```python
from build123d import *

# Parameters (mm, degrees)
BASE_EXTRUDE_DEPTH  = 20.447
CUT_EXTRUDE1_DEPTH  = 28.194
SKETCH3_W           = 5.4864
SKETCH3_H           = 1.651
BOSS_EXTRUDE1_DEPTH = 1.27


with BuildPart() as part:
    # Sketch1 → Base-Extrude (new, symmetric)
    with BuildSketch(Plane(origin=(0, 0, 0), x_dir=(1, 0, 0), z_dir=(0, 1, 0))):
        with BuildLine():
            Line((-18.4785, 20.955), (18.4785, 20.955))
            ThreePointArc((18.4785, 20.955), (24.585074162, 18.425574162), (27.1145, 12.319))
            Line((27.1145, 12.319), (27.1145, -12.319))
            ThreePointArc((27.1145, -12.319), (24.585074162, -18.425574162), (18.4785, -20.955))
            Line((18.4785, -20.955), (-18.4785, -20.955))
            ThreePointArc((-18.4785, -20.955), (-24.585074162, -18.425574162), (-27.1145, -12.319))
            Line((-27.1145, -12.319), (-27.1145, 12.319))
            ThreePointArc((-27.1145, 12.319), (-24.585074162, 18.425574162), (-18.4785, 20.955))
        make_face()
    extrude(amount=BASE_EXTRUDE_DEPTH, both=True)

    # Sketch2 → Cut-Extrude1 (cut)
    with BuildSketch(Plane.XZ.offset(20.447)):
        with BuildLine():
            Line((12.192, 20.955), (12.192, -20.955))
            Line((12.192, -20.955), (18.4785, -20.955))
            ThreePointArc((18.4785, -20.955), (24.585074162, -18.425574162), (27.1145, -12.319))
            Line((27.1145, -12.319), (27.1145, 12.319))
            ThreePointArc((27.1145, 12.319), (24.585074162, 18.425574162), (18.4785, 20.955))
            Line((18.4785, 20.955), (12.192, 20.955))
        make_face()
        with BuildLine():
            Line((-18.4785, -20.955), (-12.192, -20.955))
            Line((-12.192, -20.955), (-12.192, 20.955))
            Line((-12.192, 20.955), (-18.4785, 20.955))
            ThreePointArc((-18.4785, 20.955), (-24.585074162, 18.425574162), (-27.1145, 12.319))
            Line((-27.1145, 12.319), (-27.1145, -12.319))
            ThreePointArc((-27.1145, -12.319), (-24.585074162, -18.425574162), (-18.4785, -20.955))
        make_face()
    extrude(amount=-CUT_EXTRUDE1_DEPTH, mode=Mode.SUBTRACT)

    # Sketch3 → Boss-Extrude1 (add)
    with BuildSketch(Plane.XZ.offset(20.447)):
        with Locations((9.4488, -10.4775)):
            Rectangle(SKETCH3_W, SKETCH3_H)
        with Locations((9.4488, 10.4775)):
            Rectangle(SKETCH3_W, SKETCH3_H)
        with Locations((-9.4488, 10.4775)):
            Rectangle(SKETCH3_W, SKETCH3_H)
        with Locations((-9.4488, -10.4775)):
            Rectangle(SKETCH3_W, SKETCH3_H)
    extrude(amount=BOSS_EXTRUDE1_DEPTH)


solid = part.part
```
Geometry: final body of the model. Coordinates: model frame, mm. A direction names the side the tool comes from. Round coordinates to 2 decimals unless told otherwise and drop trailing zeros. Order: outer loops, then holes, each group sorted by start corner. A loop starts at its lowest first (then second) coordinate and runs counter-clockwise, first axis right, second up. Notation, with made-up numbers: (80, 83) -> (126, 83) arc R20 ccw to (126, 122) -> close; hole circle Ø4 at (38.25, 63). An arc over 180 degrees is marked (long way). Use one line per item in the form item = value. Start each with the question number.
1. Cut plane B-B (x = -11). Return the cut outline in (y, z) (3 decimals).
2. Draft query along Z for faces 6 (the face through (-24.65, 14.19, -18.36)), 7 (the face through (20, 7.747, 0)), 8 (the face through (-9, -21, -9.652)). Return one class per face: pulls with the +Z half, pulls with the -Z half, needs draft (parallel to the pull), parting line crosses it, or undercut.
3. Pin query (flat end, axial travel): pin 1 Ø1 at (x, y) = (10, -21) entering from -Z; pin 2 Ø19.5 at (x, z) = (3, -5.5) entering from -Y; pin 3 Ø5 at (x, z) = (0, 9.5) entering from -Y; pin 4 Ø0.6 at (x, y) = (8.5, -21) entering from +Z. Return the tip coordinate at first contact, or that it passes through.
4. Cut plane C-C (z = -1.5). Return the cut outline in (x, y).
5. Cut plane A-A (y = 15). Return the cut outline in (x, z) (1 decimal), then the cut area to 3 significant figures.
6. Reachability of faces 1 (the face through (-9, -21, 9.652)), 2 (the face through (12.192, -7, 0)), 3 (the face through (-9, -21, 11.303)), 4 (the face through (9, -21, -11.303)), 5 (the face through (-6.706, -21, 10)) from +Z, -Z, +X, -X, +Y, -Y: full face, straight path, thin tool, end or side. Return the list, or none.
7. Line query: probe 1 along X at (y, z) = (-6, 16); probe 2 along Y at (x, z) = (-9.5, 17.5); probe 3 along Y at (x, z) = (-12.5, 1.5). Output: solid intervals per line, ascending.
8. Cut plane D-D (x = -2). Return the cut outline in (y, z) (3 decimals), then the cut area to 3 significant figures.
Solution:
q1.outline = (-21.717, -11.303) -> (-20.447, -11.303) -> (-20.447, -20.955) -> (20.447, -20.955) -> (20.447, 20.955) -> (-20.447, 20.955) -> (-20.447, 11.303) -> (-21.717, 11.303) -> (-21.717, 9.652) -> (-20.447, 9.652) -> (-20.447, -9.652) -> (-21.717, -9.652) -> close
q2.face_6 = pulls with the -Z half
q2.face_7 = needs draft
q2.face_8 = undercut
q3.pin_1 = -11.3
q3.pin_2 = -21.72
q3.pin_3 = -20.45
q3.pin_4 = 11.3
q4.outline = (-27.11, 7.75) -> (-12.19, 7.75) -> (-12.19, -20.45) -> (12.19, -20.45) -> (12.19, 7.75) -> (27.11, 7.75) -> (27.11, 20.45) -> (-27.11, 20.45) -> close
q5.outline = (-27.1, -12.3) arc R8.6 ccw to (-18.5, -21) -> (18.5, -21) arc R8.6 ccw to (27.1, -12.3) -> (27.1, 12.3) arc R8.6 ccw to (18.5, 21) -> (-18.5, 21) arc R8.6 ccw to (-27.1, 12.3) -> close
q5.area = 2,210 mm^2
q6.face_1 = +X, -X, -Y
q6.face_2 = +Z, -Z, +X, -Y
q6.face_3 = +Z, +X, -X, -Y
q6.face_4 = -Z, +X, -X, -Y
q6.face_5 = +Z, -Z, -Y
q7.probe_1 = -12.19 to 12.19
q7.probe_2 = -20.45 to 20.45
q7.probe_3 = 7.75 to 20.45
q8.outline = (-20.447, -20.955) -> (20.447, -20.955) -> (20.447, 20.955) -> (-20.447, 20.955) -> close
q8.area = 1,710 mm^2
